Read the model definition and answer for the solid it produces. Units are mm, in the model's axes. A direction names the side the tool comes from. Give positions to 0.01 mm unless a question says otherwise; leave off trailing zeros. Write each loop counter-clockwise with the first axis right and the second up, starting at its lowest first coordinate (ties: lowest second). Pieces come first, ordered by that corner, then holes. Notation, with made-up numbers: M 17.5,-39 L 55.5,-39 A23 ccw 55.5,-24 Z; hole C 75.25,-34.5 d6. An arc over 180 degrees is marked long. Use a Markdown table: item, result. Add a question column.
Item 1: The mould has two halves that part along X. Classify faces 1 (the cylindrical face through (66, 2, 0)), 2 (the cylindrical face through (1.951, 2.231, 47.214)), 3 (the flat face through (-56, 2, -76)): pulls with the +X half, pulls with the -X half, needs draft (parallel to the pull), parting line crosses it, or undercut.
Item 2: For faces 4 (the flat face through (-1, 0, -2)), 5 (the flat face through (-56, 2, 76)), 6 (the flat face through (56, 2, 76)), determine the directions among +Z, -Z, +X, -X, +Y, -Y from which every point of the face is accessible in a straight line to the end or side of a thin tool.
Item 3: A cutting plane is placed at A-A on z = 71. Determine the outline of the cut face in (x, y), then the cut area to 3 significant figures.
Item 4: Given P1, Ø1.5, axis at x = -52.5, y = 2, coming from the +Z side; P2, Ø1, axis at y = 0.5, z = -13.5, coming from the +X side; P3, Ø4, axis at x = 18.75, z = 18.75, coming from the -Y side; P4, Ø3, axis at x = -52.5, z = -85, coming from the -Y side, each flat-ended and moving along its own axis, determine where each tip first touches the part or whether it passes through.
Item 5: A cutting plane is placed at B-B on y = 2.9. Count the separate pieces of the cut face and the enclosed holes in it, then the cut area to 3 significant figures.
Item 6: A cutting plane is placed at C-C on x = -29.5. Determine the outline of the cut face in (y, z), then the cut area to 3 significant figures.
Item 7: Consider probe 1 along X at (y, z) = (2.35, -66); probe 2 along X at (y, z) = (3, 18.5); probe 3 along Z at (x, y) = (-57.5, 2.9). Determine where each line is inside the solid, lowest interval first. Write a range as [from, to].
from build123d import *

# Parameters (mm, degrees)
SKETCH2_W                  = 132
SKETCH2_H                  = 232
PLATE_SIZE_DEPTH           = 4.4
SKETCH4_OUTSIDE_W          = 187.392
SKETCH4_OUTSIDE_H          = 287.392
OUTER_PROFILE_DEPTH        = 5.4
M3_CLEARANCE_HOLE1_D       = 3.5
F_18_0_18_DIAMETER_HOLE4_D = 18
M3_CLEARANCE_HOLE2_D       = 3.5
M3_CLEARANCE_HOLE3_D       = 3
M3_CLEARANCE_HOLE4_D       = 3


with BuildPart() as part:
    # Sketch2 → Plate Size (new body)
    with BuildSketch(Plane(origin=(0, 0, 0), x_dir=(1, 0, 0), z_dir=(0, 1, 0))):
        Rectangle(SKETCH2_W, SKETCH2_H)
    extrude(amount=PLATE_SIZE_DEPTH)

    # Sketch4 outside → Outer Profile (cut, through all)
    with BuildSketch(Plane(origin=(0, 0, 0), x_dir=(1, 0, 0), z_dir=(0, 1, 0))):
        Rectangle(SKETCH4_OUTSIDE_W, SKETCH4_OUTSIDE_H)
        with BuildLine():
            Line((-64.599996007, 76), (-47, 76))
            Line((-47, 76), (-47, 4))
            Line((-47, 4), (-62, 4))
            ThreePointArc((-62, 4), (-66, 0), (-62, -4))
            Line((-62, -4), (-47, -4))
            Line((-47, -4), (-47, -76))
            Line((-47, -76), (-64.599996007, -76))
            ThreePointArc((-64.599996007, -76), (-65.462483305, -76.493921289), (-65.472968926, -77.487768677))
            ThreePointArc((-65.472968926, -77.487768677), (0, -115.905117871), (65.472968926, -77.487768677))
            ThreePointArc((65.472968926, -77.487768677), (65.462483305, -76.493921289), (64.599996007, -76))
            Line((64.599996007, -76), (47, -76))
            Line((47, -76), (47, -4))
            Line((47, -4), (62, -4))
            ThreePointArc((62, -4), (66, 0), (62, 4))
            Line((62, 4), (47, 4))
            Line((47, 4), (47, 76))
            Line((47, 76), (64.599996007, 76))
            ThreePointArc((64.599996007, 76), (65.462483305, 76.493921289), (65.472968926, 77.487768677))
            ThreePointArc((65.472968926, 77.487768677), (0, 115.905117871), (-65.472968926, 77.487768677))
            ThreePointArc((-65.472968926, 77.487768677), (-65.462483305, 76.493921289), (-64.599996007, 76))
        make_face(mode=Mode.SUBTRACT)
    extrude(amount=OUTER_PROFILE_DEPTH, mode=Mode.SUBTRACT)

    # M3 Clearance Hole1 (through all)
    with Locations(Plane.XZ):
        with Locations((-55.999996141, 80.000001937), (55.999996141, 80.000001937), (-52.5, -85), (52.5, -85), (-55.999996141, 0), (55.999996141, 0)):
            Hole(M3_CLEARANCE_HOLE1_D / 2)

    # Ø18.0 (18) Diameter Hole4 (through all)
    with Locations(Plane.XZ):
        with Locations((0, -56), (0, 56)):
            Hole(F_18_0_18_DIAMETER_HOLE4_D / 2)

    # M3 Clearance Hole2 (through all)
    with Locations(Plane.XZ):
        with Locations((18.75, -18.75), (-18.75, 18.75), (18.75, 18.75), (-18.75, -18.75)):
            Hole(M3_CLEARANCE_HOLE2_D / 2)

    # M3 Clearance Hole3 (through all)
    with Locations(Plane.XZ):
        with Locations((-25.5, -66.00000008), (25.5, 65.00000008), (-25.5, 65.00000008), (25.5, -66.00000008), (-25.5, -58.00000008), (25.5, -58.00000008), (25.5, 57.00000008), (-25.5, 57.00000008)):
            Hole(M3_CLEARANCE_HOLE3_D / 2)

    # M3 Clearance Hole4 (through all)
    with Locations(Plane.XZ):
        with Locations((-20, -107), (20, -107), (-20, -82), (20, -82)):
            Hole(M3_CLEARANCE_HOLE4_D / 2)


solid = part.part
Filled in:
| question | item | result |
|---|---|---|
| 1 | face 1 | pulls with the +X half |
| 1 | face 2 | undercut |
| 1 | face 3 | needs draft |
| 2 | face 4 | +Z, -Z, +X, -X, -Y |
| 2 | face 5 | -X, +Y, -Y |
| 2 | face 6 | +X, +Y, -Y |
| 3 | outline | M -47,0 L 47,0 L 47,4.4 L -47,4.4 Z |
| 3 | area | 414 mm² |
| 4 | P1 | z = 95.19 |
| 4 | P2 | x = 47 |
| 4 | P3 | y = 0 |
| 4 | P4 | through |
| 5 | separate pieces | 1 |
| 5 | enclosed holes | 24 |
| 5 | area | 21,400 mm² |
| 6 | outline | M 0,-109.86 L 4.4,-109.86 L 4.4,109.86 L 0,109.86 Z |
| 6 | area | 967 mm² |
| 7 | probe 1 | [-47, -27], [-24, 24], [27, 47] |
| 7 | probe 2 | [-47, -20.48], [-17.02, 17.02], [20.48, 47] |
| 7 | probe 3 | [-89.06, -76], [-4, -0.9], [0.9, 4], [76, 79.1], [80.9, 89.06] |
